```python
from build123d import *

# Parameters (mm, degrees)
SKETCH1_W                = 200
SKETCH1_H                = 200
BOSS_EXTRUDE1_DEPTH      = 30
SKETCH4_W                = 175
SKETCH4_H                = 175
CUT_EXTRUDE1_DEPTH       = 30
SKETCH7_R                = 4
CUT_EXTRUDE2_DEPTH       = 210
SKETCH10_W               = 6.040230253
SKETCH10_H               = 30
BOSS_EXTRUDE2_DEPTH      = 20
SKETCH11_W               = 10
SKETCH11_H               = 30
BOSS_EXTRUDE3_DEPTH      = 20
CUT_EXTRUDE3_START       = -231
SKETCH12_R               = 4
CUT_EXTRUDE3_DEPTH       = 231
SKETCH13_R               = 4
CUT_EXTRUDE5_DEPTH       = 231
SKETCH14_R               = 4
CUT_EXTRUDE6_DEPTH       = 250.5
SKETCH15_R               = 30
SKETCH15_R_2             = 22
BOSS_EXTRUDE5_DEPTH      = 201
SKETCH17_R               = 22
CUT_EXTRUDE7_DEPTH       = 201
SKETCH21_W               = 9.5
SKETCH21_H               = 28.855904386
BOSS_EXTRUDE6_DEPTH      = 26
SKETCH22_W               = 9.5
SKETCH22_H               = 6.040230253
CUT_EXTRUDE10_DEPTH      = 49
SKETCH23_W               = 10.008922512
SKETCH23_H               = 28.855904386
BOSS_EXTRUDE7_DEPTH      = 21
SKETCH24_W               = 9.5
SKETCH24_H               = 1.144095614
CUT_EXTRUDE11_DEPTH      = 27
SKETCH26_W               = 0.50137975
SKETCH26_H               = 20.893624798
CUT_EXTRUDE12_DEPTH      = 35
SKETCH27_R               = 49.192783102
CUT_EXTRUDE13_DEPTH      = 175
SKETCH28_R               = 41.209023923
CUT_EXTRUDE14_DEPTH      = 175
CUT_EXTRUDE15_DEPTH      = 246.814971066
CUT_EXTRUDE15_DEPTH_BACK = 210


with BuildPart() as part:
    # Sketch1 → Boss-Extrude1 (new body)
    with BuildSketch(Plane(origin=(0, 0, 0), x_dir=(1, 0, 0), z_dir=(0, 1, 0))):
        Rectangle(SKETCH1_W, SKETCH1_H)
    extrude(amount=BOSS_EXTRUDE1_DEPTH)

    # Sketch4 → Cut-Extrude1 (cut)
    with BuildSketch(Plane(origin=(0, 30, 0), x_dir=(1, 0, 0), z_dir=(0, 1, 0))):
        Rectangle(SKETCH4_W, SKETCH4_H)
    extrude(amount=-CUT_EXTRUDE1_DEPTH, mode=Mode.SUBTRACT)

    # Sketch7 → Cut-Extrude2 (cut)
    with BuildSketch(Plane.ZY.offset(100)):
        with Locations((0, 15)):
            Circle(SKETCH7_R)
    extrude(amount=-CUT_EXTRUDE2_DEPTH, mode=Mode.SUBTRACT)

    # Sketch10 → Boss-Extrude2 (add)
    with BuildSketch(Plane.ZY.offset(100)):
        with Locations((-11.64671233, 15)):
            Rectangle(SKETCH10_W, SKETCH10_H)
    extrude(amount=BOSS_EXTRUDE2_DEPTH)

    # Sketch11 → Boss-Extrude3 (add)
    with BuildSketch(Plane.XY.offset(-8.626597203)):
        with Locations((-115, 15)):
            Rectangle(SKETCH11_W, SKETCH11_H)
    extrude(amount=BOSS_EXTRUDE3_DEPTH)

    # Sketch12 → Cut-Extrude3 (cut)
    with BuildSketch(Plane(origin=(100, 0, 0), x_dir=(0, 0, -1), z_dir=(1, 0, 0)).offset(CUT_EXTRUDE3_START)):
        with Locations(Location((0, 15, 0), (0, 0, 180))):
            Circle(SKETCH12_R)
    extrude(amount=CUT_EXTRUDE3_DEPTH, mode=Mode.SUBTRACT)

    # Sketch13 → Cut-Extrude5 (cut)
    with BuildSketch(Plane(origin=(0, 30, 0), x_dir=(1, 0, 0), z_dir=(0, 1, 0))):
        with Locations(Location((-93.69452155, -93.045501349, 0), (0, 0, 270))):
            Circle(SKETCH13_R)
    extrude(amount=-CUT_EXTRUDE5_DEPTH, mode=Mode.SUBTRACT)

    # Sketch14 → Cut-Extrude6 (cut)
    with BuildSketch(Plane.XY.offset(100)):
        with Locations((0, 13.614739596)):
            Circle(SKETCH14_R)
    extrude(amount=-CUT_EXTRUDE6_DEPTH, mode=Mode.SUBTRACT)

    # Sketch15 → Boss-Extrude5 (add)
    with BuildSketch(Plane(origin=(100, 0, 0), x_dir=(0, 0, -1), z_dir=(1, 0, 0))):
        with Locations((0, 15)):
            Circle(SKETCH15_R)
        with Locations((0, 15)):
            Circle(SKETCH15_R_2, mode=Mode.SUBTRACT)
    extrude(amount=-BOSS_EXTRUDE5_DEPTH)

    # Sketch17 → Cut-Extrude7 (cut)
    with BuildSketch(Plane(origin=(100, 0, 0), x_dir=(0, 0, -1), z_dir=(1, 0, 0))):
        with Locations((0.074377339, 15.100772812)):
            Circle(SKETCH17_R)
    extrude(amount=-CUT_EXTRUDE7_DEPTH, mode=Mode.SUBTRACT)


with BuildPart() as cut_extrude7_piece_1:
    # of the separate pieces the step leaves, piece 1, a body of its own (cut_extrude7_pieces)
    add(part.part.solids().sort_by_distance((-100, 0, -100))[0])



with BuildPart() as cut_extrude7_piece_2:
    # of the separate pieces the step leaves, piece 2, a body of its own (cut_extrude7_pieces)
    add(part.part.solids().sort_by_distance((-101, 0, -14.666827456))[0])

    # Sketch21 → Boss-Extrude6 (add)
    with BuildSketch(Plane(origin=(0, 0, -14.666827456), x_dir=(-1, 0, 0), z_dir=(0, 0, -1))):
        with Locations((115.25, 15.572047807)):
            Rectangle(SKETCH21_W, SKETCH21_H)
    extrude(amount=BOSS_EXTRUDE6_DEPTH)

    # Sketch22 → Cut-Extrude10 (cut)
    with BuildSketch(Plane(origin=(0, 30, 0), x_dir=(1, 0, 0), z_dir=(0, 1, 0))):
        with Locations((-105.75, 11.64671233)):
            Rectangle(SKETCH22_W, SKETCH22_H)
    extrude(amount=-CUT_EXTRUDE10_DEPTH, mode=Mode.SUBTRACT)


with BuildPart() as cut_extrude7_piece_1_1:
    add(cut_extrude7_piece_1.part)

    add(cut_extrude7_piece_2.part)  # Boss-Extrude7 merges Cut-Extrude7 piece 2
    # Sketch23 → Boss-Extrude7 (add)
    with BuildSketch(Plane(origin=(-110.5, 0, 0), x_dir=(0, 0, -1), z_dir=(1, 0, 0))):
        with Locations((35.6623662, 15.572047807)):
            Rectangle(SKETCH23_W, SKETCH23_H)
    extrude(amount=BOSS_EXTRUDE7_DEPTH)

    # Sketch24 → Cut-Extrude11 (cut)
    with BuildSketch(Plane(origin=(0, 0, -14.666827456), x_dir=(-1, 0, 0), z_dir=(0, 0, -1))):
        with Locations((115.25, 0.572047807)):
            Rectangle(SKETCH24_W, SKETCH24_H)
    extrude(amount=-CUT_EXTRUDE11_DEPTH, mode=Mode.SUBTRACT)

    # Sketch26 → Cut-Extrude12 (cut)
    with BuildSketch(Plane.XZ):
        with Locations((-110.249310125, 1.820215196)):
            Rectangle(SKETCH26_W, SKETCH26_H)
    extrude(amount=-CUT_EXTRUDE12_DEPTH, mode=Mode.SUBTRACT)

    # Sketch27 → Cut-Extrude13 (cut)
    with BuildSketch(Plane(origin=(-87.5, 0, 0), x_dir=(0, 0, -1), z_dir=(1, 0, 0))):
        with Locations((-31.916352411, 15.376133278)):
            Circle(SKETCH27_R)
    extrude(amount=CUT_EXTRUDE13_DEPTH, mode=Mode.SUBTRACT)

    # Sketch28 → Cut-Extrude14 (cut)
    with BuildSketch(Plane(origin=(-87.5, 0, 0), x_dir=(0, 0, -1), z_dir=(1, 0, 0))):
        with Locations((37.762434774, 15.494435184)):
            Circle(SKETCH28_R)
    extrude(amount=CUT_EXTRUDE14_DEPTH, mode=Mode.SUBTRACT)

    # Sketch30 → Cut-Extrude15 (cut, two sides: drawn at the far end of the back side and taken through both)
    with BuildSketch(Plane(origin=(100, 0, 0), x_dir=(0, 0, -1), z_dir=(1, 0, 0)).offset(-CUT_EXTRUDE15_DEPTH_BACK)):
        with BuildLine():
            Line((-112.795739645, -240.367951942), (25.980762114, 0))
            ThreePointArc((25.980762114, 0), (30, 15), (25.980762114, 30))
            Line((25.980762114, 30), (-112.795739645, 270.367951942))
            Line((-112.795739645, 270.367951942), (-667.901746678, 270.367951942))
            Line((-667.901746678, 270.367951942), (-667.901746678, -240.367951942))
            Line((-667.901746678, -240.367951942), (-112.795739645, -240.367951942))
        make_face()
    extrude(amount=CUT_EXTRUDE15_DEPTH + CUT_EXTRUDE15_DEPTH_BACK, mode=Mode.SUBTRACT)


solid = cut_extrude7_piece_1_1.part
```
Geometry check sheet. Reference: the model listing, model coordinates, mm. A direction names the side the tool comes from. Give positions to 0.01 mm unless a question says otherwise; leave off trailing zeros. Loops run counter-clockwise (first coordinate to the right, second up) from the corner with the lowest first, then second, coordinate; pieces in that order, holes last. Notation, with made-up numbers: M 73,17 L 126,17 A21 cw 126,50 Z; hole C 76,40.25 d4. An arc over 180 degrees is marked long. Answer as CSV lines item,"result".
Item 1: Cross-section at B-B on x = 0. Record the cut outline in (y, z).
Values:
outline,"M 0,-100 L 9.61,-100 L 9.61,-87.5 L 0,-87.5 Z; M 17.61,-100 L 30,-100 L 30,-87.5 L 17.61,-87.5 Z"
Item 2: Cross-section at A-A on z = 0. Record the cut outline in (x, y), and give its area (3 significant figures).
Values:
outline,"M -120,1.14 L -110.5,1.14 L -110.5,11 L -120,11 Z; M -120,19 L -110.5,19 L -110.5,30 L -120,30 Z"
area,"198 mm²"
Item 3: Cross-section at D-D on x = -102. Record the cut outline in (y, z), and give its area (3 significant figures).
Values:
outline,"M 1.14,-40.67 L 30,-40.67 L 30,-30.66 L 1.14,-30.66 Z"
area,"289 mm²"
Item 4: Access from +Z, -Z, +X, -X, +Y, -Y to the whole of each face (thin tool, end or side, straight path). Record for faces 4 (the flat face through (-110, 15, -40.667)), 5 (the flat face through (-105, 15, -30.658)), 6 (the cylindrical face through (-94, 15, -30)).
Values:
face 4,"-Z, -X, +Y, -Y"
face 5,"+Z, +Y, -Y"
face 6,"+Z, +X"
Item 5: Depth check by flat-ended pin: P1, Ø1, axis at x = -93.5, y = 17.5, coming from the +Z side; P2, Ø5, axis at x = -105.5, y = 17.5, coming from the +Z side; P3, Ø22, axis at x = -113, z = -25, coming from the -Y side. Enter the tip coordinate at first touch or a pass-through.
Values:
P1,"stops at z = -29.85"
P2,"stops at z = -30.66"
P3,"stops at y = 1.14"
Item 6: Release check for a two-part mould opening along X. For faces 1 (the cylindrical face through (94, 15, -30)), 2 (the flat face through (87.5, 15, -56)), 3 (the flat face through (-120, 15, -14)) record: pulls with the +X half, pulls with the -X half, needs draft (parallel to the pull), parting line crosses it, or undercut.
Values:
face 1,"needs draft"
face 2,"undercut"
face 3,"pulls with the -X half"
Item 7: Cross-section at C-C on y = 5.5. Record the cut outline in (x, z).
Values:
outline,"M -120,-40.67 L -100,-40.67 L -100,-100 L 100,-100 L 100,-28.46 L 87.5,-28.46 L 87.5,-87.5 L -87.5,-87.5 L -87.5,-28.46 L -100,-28.46 L -100,-30.66 L -110.5,-30.66 L -110.5,11.37 L -120,11.37 Z"
Item 8: Material ranges on line 1 (Y direction, x = -117, z = 0); line 2 (Y direction, x = 0, z = -96.5); line 3 (X direction, y = 9.5, z = -75), recorded low to high.
Values:
line 1,"y = 1.14 to 11, 19 to 30"
line 2,"y = 0 to 9.61, 17.61 to 30"
line 3,"x = -100 to -87.5, 87.5 to 100"
